Can you work these out from the model? Positions are in its coordinate system, mm. A direction names the side the tool comes from. Round coordinates to 2 decimals unless told otherwise and drop trailing zeros. Order: outer loops, then holes, each group sorted by start corner. A loop starts at its lowest first (then second) coordinate and runs counter-clockwise, first axis right, second up. Notation, with made-up numbers: (52, 41.5) -> (59, 41.5) arc R15 cw to (59, 55.5) -> close; hole circle Ø2 at (-18.75, -24). An arc over 180 degrees is marked (long way). Use a Markdown table: item, result. Add a question column.
Q1. I need wall thicknesses on line 1 along Z through (x, y) = (32.15, 26.5); line 2 along X through (y, z) = (13.75, 41.5); line 3 along X through (y, z) = (13.5, -19). Which ranges of each line are inside material? Lowest first, please. Write a range as [from, to].
Q2. I'm going to push flat-ended pins straight in: pin 1 Ø1.5 at (x, z) = (-21, 34.5) entering from +Y; pin 2 Ø1.5 at (x, z) = (24.5, 19) entering from +Y. Where does each tip first touch, or does it pass through?
Q3. If we section it at B-B on x = -1: List the corners of the cut face in (y, z) for me, plus the area to 3 significant figures.
Q4. We'd pull the mould along X, two halves only. Please class faces 1 (the face through (3, 8.85, 43)), 2 (the face through (22, 27, -43)), 3 (the face through (-32.972, 27.987, -10.445)): +X half, -X half, draft (parallel to the pull), parting line (faces both ways), or undercut.
Q5. If we section it at A-A on z = 10.25: List the corners of the cut face in (x, y) for me.
Q6. If we section it at D-D on y = 15.75: List the corners of the cut face in (x, z) for me, plus the area to 4 significant figures.
Q7. For faces 4 (the face through (0, 4, -1)), 5 (the face through (-25, 25, -43)), 6 (the face through (15, 24, -43)), which set-ups out of +Z, -Z, +X, -X, +Y, -Y let a thin tool reach every point of the face, with its end or its side?
Q8. If we section it at C-C on y = 21.5: List the corners of the cut face in (x, z) for me, plus the area to 3 significant figures.
```python
from build123d import *

# Parameters (mm, degrees)
SKETCH1_W               = 70
SKETCH1_H               = 90
BOSS_EXTRUDE1_DEPTH     = 30
SHELL1_T                = -4
SKETCH2_W               = 13.25
SKETCH2_H               = 11.5
SKETCH2_W_2             = 11.25
SKETCH2_H_2             = 9.5
CUT_EXTRUDE1_DEPTH      = 7
SKETCH3_W               = 18
SKETCH3_H               = 10
CUT_EXTRUDE2_DEPTH      = 7
SKETCH4_W               = 15
SKETCH4_H               = 6
CUT_EXTRUDE3_DEPTH      = 7
SKETCH6_R               = 4
SKETCH6_R_2             = 1.5
BOSS_EXTRUDE2_DEPTH     = 7
CUT_EXTRUDE4_DEPTH      = 86.32877592
CUT_EXTRUDE4_DEPTH_BACK = 86.32877592
SKETCH7_R               = 1.5
SKETCH8_W               = 10
SKETCH8_H               = 4
CUT_EXTRUDE5_DEPTH      = 7


with BuildPart() as part:
    # Sketch1 → Boss-Extrude1 (new body)
    with BuildSketch(Plane(origin=(0, 0, 0), x_dir=(1, 0, 0), z_dir=(0, 1, 0))):
        Rectangle(SKETCH1_W, SKETCH1_H)
    extrude(amount=BOSS_EXTRUDE1_DEPTH)

    # Shell1
    shell1_openings = [part.faces().sort_by_distance(p)[0] for p in [
        (0, 30, 0),
    ]]
    offset(amount=SHELL1_T, openings=shell1_openings, kind=Kind.INTERSECTION)

    # Sketch2 → Cut-Extrude1 (cut)
    # profile 1 of 2: a face of its own
    with BuildSketch(Plane.XY.offset(45)):
        with Locations((-12.349103725, 13.85)):
            Rectangle(SKETCH2_W, SKETCH2_H)
        with Locations((-12.349103725, 13.85)):
            Rectangle(SKETCH2_W_2, SKETCH2_H_2, mode=Mode.SUBTRACT)
    # profile 2 of 2: a face of its own
    with BuildSketch(Plane.XY.offset(45)):
        with Locations((-12.349103725, 13.85)):
            Rectangle(SKETCH2_W_2, SKETCH2_H_2)
    extrude(amount=-CUT_EXTRUDE1_DEPTH, mode=Mode.SUBTRACT)

    # Sketch3 → Cut-Extrude2 (cut)
    with BuildSketch(Plane.XY.offset(45)):
        with Locations((2.275896275, 13.85)):
            Rectangle(SKETCH3_W, SKETCH3_H)
    extrude(amount=-CUT_EXTRUDE2_DEPTH, mode=Mode.SUBTRACT)

    # Sketch4 → Cut-Extrude3 (cut)
    with BuildSketch(Plane(origin=(0, 0, -45), x_dir=(-1, 0, 0), z_dir=(0, 0, -1))):
        with Locations((-14.5, 27)):
            Rectangle(SKETCH4_W, SKETCH4_H)
    extrude(amount=-CUT_EXTRUDE3_DEPTH, mode=Mode.SUBTRACT)

    # Sketch6 → Boss-Extrude2 (add)
    # profile 1 of 4: a face of its own
    with BuildSketch(Plane(origin=(0, 0, -1.719487256), x_dir=(1, 0, 0), z_dir=(0, -1, 0))):
        with Locations(Location((-24.474103725, 19.735790835, 0), (0, 0, 270))):
            Circle(SKETCH6_R)
        with Locations(Location((-24.474103725, 19.735790835, 0), (0, 0, 270))):
            Circle(SKETCH6_R_2, mode=Mode.SUBTRACT)
    # profile 2 of 4: a face of its own
    with BuildSketch(Plane(origin=(0, 0, -1.719487256), x_dir=(1, 0, 0), z_dir=(0, -1, 0))):
        with Locations(Location((25.025896275, 19.735790835, 0), (0, 0, 270))):
            Circle(SKETCH6_R)
        with Locations(Location((25.025896275, 19.735790835, 0), (0, 0, 270))):
            Circle(SKETCH6_R_2, mode=Mode.SUBTRACT)
    # profile 3 of 4: a face of its own
    with BuildSketch(Plane(origin=(0, 0, -1.719487256), x_dir=(1, 0, 0), z_dir=(0, -1, 0))):
        with Locations(Location((20.309236753, -34.964209165, 0), (0, 0, 270))):
            Circle(SKETCH6_R)
        with Locations(Location((20.309236753, -34.964209165, 0), (0, 0, 270))):
            Circle(SKETCH6_R_2, mode=Mode.SUBTRACT)
    # profile 4 of 4: a face of its own
    with BuildSketch(Plane(origin=(0, 0, -1.719487256), x_dir=(1, 0, 0), z_dir=(0, -1, 0))):
        with Locations(Location((-7.207089355, -34.964209165, 0), (0, 0, 270))):
            Circle(SKETCH6_R)
        with Locations(Location((-7.207089355, -34.964209165, 0), (0, 0, 270))):
            Circle(SKETCH6_R_2, mode=Mode.SUBTRACT)
    extrude(amount=-BOSS_EXTRUDE2_DEPTH)

    # Sketch7 → Cut-Extrude4 (cut, two sides: drawn at the far end of the back side and taken through both)
    with BuildSketch(Plane.ZY.offset(-31).offset(-CUT_EXTRUDE4_DEPTH_BACK)):
        with Locations((-30.75, 26.5)):
            Circle(SKETCH7_R)
        with Locations((-10.25, 26.5)):
            Circle(SKETCH7_R)
        with Locations((10.25, 26.5)):
            Circle(SKETCH7_R)
        with Locations((30.75, 26.5)):
            Circle(SKETCH7_R)
    extrude(amount=CUT_EXTRUDE4_DEPTH + CUT_EXTRUDE4_DEPTH_BACK, mode=Mode.SUBTRACT)

    # Sketch8 → Cut-Extrude5 (cut)
    with BuildSketch(Plane(origin=(0, 0, -45), x_dir=(-1, 0, 0), z_dir=(0, 0, -1))):
        with Locations((20, 25)):
            Rectangle(SKETCH8_W, SKETCH8_H)
    extrude(amount=-CUT_EXTRUDE5_DEPTH, mode=Mode.SUBTRACT)


solid = part.part
```
Answer below:
| question | item | result |
|---|---|---|
| 1 | line 1 | [-45, -32.25], [-29.25, -11.75], [-8.75, 8.75], [11.75, 29.25], [32.25, 45] |
| 1 | line 2 | [-35, -18.97], [11.28, 35] |
| 1 | line 3 | [-35, -31], [31, 35] |
| 2 | pin 1 | y = 4 |
| 2 | pin 2 | y = 7 |
| 3 | outline | (0, -45) -> (30, -45) -> (30, -41) -> (4, -41) -> (4, 41) -> (8.85, 41) -> (8.85, 45) -> (0, 45) -> close; (18.85, 41) -> (30, 41) -> (30, 45) -> (18.85, 45) -> close |
| 3 | area | 528 mm² |
| 4 | face 1 | undercut |
| 4 | face 2 | undercut |
| 4 | face 3 | draft |
| 5 | outline | (-35, 0) -> (35, 0) -> (35, 25) -> (31, 25) -> (31, 4) -> (-31, 4) -> (-31, 25) -> (-35, 25) -> close; (-35, 28) -> (-31, 28) -> (-31, 30) -> (-35, 30) -> close; (31, 28) -> (35, 28) -> (35, 30) -> (31, 30) -> close |
| 6 | outline | (-35, -45) -> (35, -45) -> (35, 45) -> (11.28, 45) -> (11.28, 41) -> (31, 41) -> (31, -41) -> (-31, -41) -> (-31, 41) -> (-18.97, 41) -> (-18.97, 45) -> (-35, 45) -> close |
| 6 | area | 1,095 mm² |
| 7 | face 4 | +Y |
| 7 | face 5 | -Z |
| 7 | face 6 | -Z, +Y |
| 8 | outline | (-35, -45) -> (35, -45) -> (35, 45) -> (-35, 45) -> close; hole (-31, -41) -> (31, -41) -> (31, 41) -> (-31, 41) -> close |
| 8 | area | 1,220 mm² |
